Verification items for the finished model (mm, model axes). Round coordinates to 2 decimals unless told otherwise and drop trailing zeros. Write each loop counter-clockwise with the first axis right and the second up, starting at its lowest first coordinate (ties: lowest second). Pieces come first, ordered by that corner, then holes. Notation, with made-up numbers: M 43,85 L 99,85 A11 ccw 99,102 Z; hole C 50.5,85 d7. An arc over 180 degrees is marked long. Answer in a Markdown table with one row per item. Add a question column.
1. Go/stop test with flat-tipped pins: pin 1 Ø2 at (x, y) = (-28, 52) entering from -Z; pin 2 Ø3 at (y, z) = (18.5, -36.5) entering from +X; pin 3 Ø12 at (x, z) = (-21, -35) entering from +Y; pin 4 Ø1 at (y, z) = (59.5, 33) entering from -X. Record where each tip stops, or that it passes through.
2. Draft check along X on faces 1 (the cylindrical face through (-10.189, 85.871, 45.882)), 2 (the cylindrical face through (45.877, 152.708, -14.225)), 3 (the cylindrical face through (-10.84, 87.49, 48.81)), 4 (the flat face through (-34, 0, 33)). Enter one of: pulls with the +X half, pulls with the -X half, needs draft (parallel to the pull), parting line crosses it, or undercut.
3. Material ranges on probe 1 along X at (y, z) = (159, 1.5); probe 2 along Z at (x, y) = (0, 84); probe 3 along X at (y, z) = (43.5, 11) (3 decimals), recorded low to high.
4. Sectioned sample at B-B on y = 55.5. Record the cut outline in (x, z).
5. Sectioned sample at C-C on x = 10.5. Record the cut outline in (y, z).
6. Sectioned sample at A-A on x = 33.5. Record the cut outline in (y, z), plus the area to 3 significant figures.
```python
from build123d import *

# Parameters (mm, degrees)
EXTRUDE_1_OUTLINE_R      = 50
EXTRUDE_1_OUTLINE_R_2    = 47
EXTRUDE_1_DEPTH          = 200
CUT_EXTRUDE_1_DEPTH      = 213.132034356
CUT_EXTRUDE_1_DEPTH_BACK = 213.132034356
SKETCH_2_R               = 65.5


# Read off the part's stored shape, not the designer's step: Вытянуть-Тонкостенный1
with BuildPart() as part:
    # Вытянуть-Тонкостенный1 outline → Вытянуть-Тонкостенный1 (new body)
    with BuildSketch(Plane(origin=(0, 0, 0), x_dir=(1, 0, 0), z_dir=(0, 1, 0))):
        Circle(EXTRUDE_1_OUTLINE_R)
        Circle(EXTRUDE_1_OUTLINE_R_2, mode=Mode.SUBTRACT)
    extrude(amount=EXTRUDE_1_DEPTH)

    # Эскиз2 → Вырез-Вытянуть1 (cut, two sides: drawn at the far end of the back side and taken through both)
    with BuildSketch(Plane(origin=(0, 0, 0), x_dir=(1, 0, 0), z_dir=(0, -0.5735764363510444, -0.819152044288993)).offset(-CUT_EXTRUDE_1_DEPTH_BACK)):
        with Locations((0, -180)):
            Circle(SKETCH_2_R)
    extrude(amount=CUT_EXTRUDE_1_DEPTH + CUT_EXTRUDE_1_DEPTH_BACK, mode=Mode.SUBTRACT)


solid = part.part
```
Geometry check:
| question | item | result |
|---|---|---|
| 1 | pin 1 | stops at z = -42.08 |
| 1 | pin 2 | stops at x = 35.71 |
| 1 | pin 3 | passes through |
| 1 | pin 4 | stops at x = -38 |
| 2 | face 1 | undercut |
| 2 | face 2 | undercut |
| 2 | face 3 | parting line crosses it |
| 2 | face 4 | needs draft |
| 3 | probe 1 | x = -49.98 to -46.98, 46.98 to 49.98 |
| 3 | probe 2 | z = -50 to -47, 47 to 50 |
| 3 | probe 3 | x = -48.775 to -45.695, 45.695 to 48.775 |
| 4 | outline | C 0,0 d100; hole C 0,0 d94 |
| 5 | outline | M 0,-48.89 L 106.58,-48.89 L 108.73,-45.81 L 0,-45.81 Z; M 0,45.81 L 172.89,45.81 L 175.04,48.89 L 0,48.89 Z |
| 6 | outline | M 0,-37.12 L 125.04,-37.12 L 127.95,-32.97 L 0,-32.97 Z; M 0,32.97 L 174.11,32.97 L 177.02,37.12 L 0,37.12 Z |
| 6 | area | 1,250 mm2 |
